Geometry: final body of the model. Coordinates: model frame, mm. Coordinates: 2 decimals unless noted, no trailing zeros. Order: outer loops, then holes, each group sorted by start corner. A loop starts at its lowest first (then second) coordinate and runs counter-clockwise, first axis right, second up. Notation, with made-up numbers: (79.25, 75) -> (124.25, 75) arc R13 ccw to (124.25, 84) -> close; hole circle Ø10 at (51, 40). An arc over 180 degrees is marked (long way). Answer in a Markdown table with one row per item. Add a question column.
1) Section query D-D on z = -3.5. Return the cut outline in (x, y) (3 decimals), then the cut area to 3 significant figures.
2) Ray query, line 1 (X direction, y = 2.9, z = 67); line 2 (Z direction, x = -2, y = 1.8); line 3 (Z direction, x = 25, y = 2.1). Return the intervals inside material, ascending. Write a range as from..to.
3) Section query B-B on x = 15. Return the cut outline in (y, z).
4) Section query C-C on x = 25. Return the cut outline in (y, z).
5) Section query A-A on z = -70. Return the cut outline in (x, y).
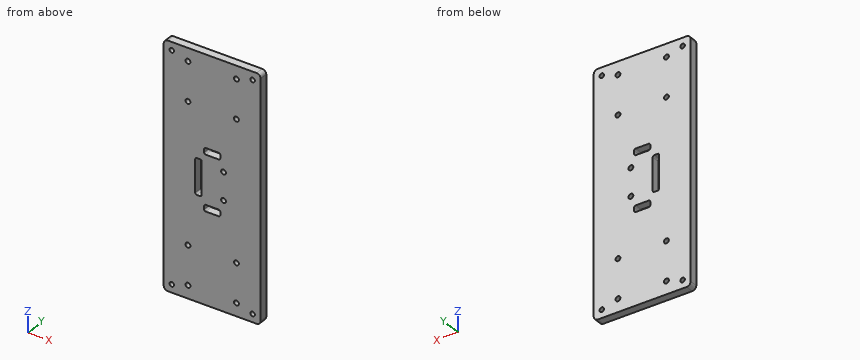
Autodesk Inventor part; units mm, degrees
ref_plane "YZ Plane" through (0, 0, 0) normal (1, 0, 0) x (0, 1, 0)
ref_plane "XZ Plane" through (0, 0, 0) normal (0, 1, 0) x (-1, 0, 0)
ref_plane "XY Plane" through (0, 0, 0) normal (0, 0, 1) x (1, 0, 0)
sketch "Sketch1" plane through (0, 0, 0) normal (0, 1, 0) x (-1, 0, 0)
  line L0 (-30, 75) -> (30, 75)
  line L1 (30, 75) -> (30, -75)
  line L2 (30, -75) -> (-30, -75)
  line L3 (-30, -75) -> (-30, 75)
  line L4 (30, 75) -> (25, 75)
  line L5 (25, 75) -> (25, 70)
  line L6 (25, 70) -> (30, 70)
  line L7 (30, 70) -> (30, 75)
  line L8 (-30, 75) -> (-25, 75)
  line L9 (-25, 75) -> (-25, 70)
  line L10 (-25, 70) -> (-30, 70)
  line L11 (-30, 70) -> (-30, 75)
  line L12 (30, -75) -> (25, -75)
  line L13 (25, -75) -> (25, -70)
  line L14 (25, -70) -> (30, -70)
  line L15 (30, -70) -> (30, -75)
  line L16 (-30, -75) -> (-25, -75)
  line L17 (-25, -75) -> (-25, -70)
  line L18 (-25, -70) -> (-30, -70)
  line L19 (-30, -70) -> (-30, -75)
  circle A0 centre (25, 70) radius 1.4
  circle A1 centre (-25, 70) radius 1.4
  circle A2 centre (25, -70) radius 1.4
  circle A3 centre (-25, -70) radius 1.4
  line L20 (0, 75) -> (13, 75)
  line L21 (0, 75) -> (-13, 75)
  line L22 (-9.515, 11.025) -> (9.515, 11.025)
  line L23 (9.515, 11.025) -> (9.515, -11.025)
  line L24 (9.515, -11.025) -> (-9.515, -11.025)
  line L25 (-9.515, -11.025) -> (-9.515, 11.025)
  line L26 (-9.515, 11.025) -> (9.515, -11.025) construction
  line L27 (9.515, 11.025) -> (-9.515, -11.025) construction
  line L28 (-9.515, -11.025) -> (-7.015, -11.025)
  line L29 (-7.015, -11.025) -> (-7.015, -8.525)
  line L30 (-7.015, -8.525) -> (-9.515, -8.525)
  line L31 (-9.515, -8.525) -> (-9.515, -11.025)
  line L32 (-9.515, 11.025) -> (-7.015, 11.025)
  line L33 (-7.015, 11.025) -> (-7.015, 8.525)
  line L34 (-7.015, 8.525) -> (-9.515, 8.525)
  line L35 (-9.515, 8.525) -> (-9.515, 11.025)
  circle A4 centre (-7.015, 8.525) radius 1.5
  circle A5 centre (-7.015, -8.525) radius 1.5
  line L36 (9.515, 0) -> (8.515, 0)
  line L37 (6.515, -11.025) -> (10.515, -11.025)
  line L38 (10.515, -11.025) -> (10.515, 11.025)
  line L39 (10.515, 11.025) -> (6.515, 11.025)
  line L40 (6.515, 11.025) -> (6.515, -11.025)
  line L41 (6.515, -11.025) -> (10.515, 11.025) construction
  line L42 (10.515, -11.025) -> (6.515, 11.025) construction
  line L43 (0, -75) -> (-20, -75)
  line L44 (-20, -75) -> (-20, -35)
  line L45 (-20, -35) -> (0, -35)
  line L46 (0, -35) -> (0, -75)
  line L47 (0, -75) -> (20, -75)
  line L48 (20, -75) -> (20, -35)
  line L49 (20, -35) -> (0, -35)
  line L50 (0, -35) -> (0, -75)
  line L51 (0, 75) -> (-20, 75)
  line L52 (-20, 75) -> (-20, 35)
  line L53 (-20, 35) -> (0, 35)
  line L54 (0, 35) -> (0, 75)
  line L55 (0, 35) -> (20, 35)
  line L56 (20, 35) -> (20, 75)
  line L57 (20, 75) -> (0, 75)
  line L58 (0, 75) -> (0, 35)
  line L59 (-20, -35) -> (20, -35)
  line L60 (20, -35) -> (20, -43)
  line L61 (20, -43) -> (-20, -43)
  line L62 (-20, -43) -> (-20, -35)
  line L63 (-20, 35) -> (20, 35)
  line L64 (20, 35) -> (20, 43)
  line L65 (20, 43) -> (-20, 43)
  line L66 (-20, 43) -> (-20, 35)
  line L67 (-20, 43) -> (-15, 43)
  line L68 (-15, 43) -> (15, 43)
  line L69 (15, 43) -> (15, 67)
  line L70 (15, 67) -> (-15, 67)
  line L71 (-15, 67) -> (-15, 43)
  line L72 (0, -43) -> (-15, -43)
  line L73 (15, -43) -> (15, -67)
  line L74 (15, -67) -> (-15, -67)
  line L75 (-15, -67) -> (-15, -43)
  circle A6 centre (-15, -67) radius 1.5
  circle A7 centre (15, -67) radius 1.5
  circle A8 centre (-15, -43) radius 1.5
  circle A9 centre (15, -43) radius 1.5
  circle A10 centre (-15, 67) radius 1.5
  circle A11 centre (-15, 43) radius 1.5
  circle A12 centre (15, 43) radius 1.5
  circle A13 centre (15, 67) radius 1.5
  line L76 (-20, 35) -> (20, 35)
  line L77 (20, 35) -> (20, 19)
  line L78 (20, 19) -> (-20, 19)
  line L79 (-20, 19) -> (-20, 35)
  line L80 (20, -35) -> (-20, -35)
  line L81 (-20, -35) -> (-20, -19)
  line L82 (-20, -19) -> (20, -19)
  line L83 (20, -19) -> (20, -35)
  line L84 (0, 19) -> (5, 19)
  line L85 (5, 19) -> (5, 15)
  line L86 (5, 15) -> (0, 15)
  line L87 (0, 15) -> (0, 19)
  line L88 (0, 19) -> (-5, 19)
  line L89 (-5, 19) -> (-5, 15)
  line L90 (-5, 15) -> (0, 15)
  line L91 (0, 15) -> (0, 19)
  line L92 (0, -19) -> (5, -19)
  line L93 (5, -19) -> (5, -15)
  line L94 (5, -15) -> (0, -15)
  line L95 (0, -15) -> (0, -19)
  line L96 (0, -15) -> (-5, -15)
  line L97 (-5, -15) -> (-5, -19)
  line L98 (-5, -19) -> (0, -19)
  line L99 (0, -19) -> (0, -15)
  point P0 (0, 0)
  point P1 (6.515, 11.025)
  point P2 (6.515, -11.025)
  point P3 (-5, 19)
  point P4 (5, 19)
  point P5 (0, 15)
  dimension "d0" = 60
  dimension "d1" = 150
  dimension "d2" = 5
  dimension "d3" = 5
  dimension "d4" = 5
  dimension "d5" = 5
  dimension "d6" = 5
  dimension "d7" = 5
  dimension "d8" = 5
  dimension "d9" = 5
  dimension "d10" = 2.8
  dimension "d11" = 2.8
  dimension "d39" = 19.03
  dimension "d40" = 22.05
  dimension "d41" = 2.5
  dimension "d42" = 2.5
  dimension "d43" = 2.5
  dimension "d44" = 2.5
  dimension "d45" = 3
  dimension "d46" = 3
  dimension "d47" = 1
  dimension "d48" = 4
  dimension "d54" = 20
  dimension "d55" = 40
  dimension "d56" = 20
  dimension "d57" = 20
  dimension "d58" = 40
  dimension "d59" = 20
  dimension "d60" = 8
  dimension "d61" = 8
  dimension "d62" = 5
  dimension "d63" = 30
  dimension "d64" = 24
  dimension "d65" = 24
  dimension "d66" = 3
  dimension "d67" = 3
  dimension "d68" = 3
  dimension "d69" = 3
  dimension "d70" = 3
  dimension "d71" = 3
  dimension "d72" = 3
  dimension "d75" = 16
  dimension "d76" = 16
  dimension "d77" = 5
  dimension "d78" = 4
  dimension "d79" = 5
  dimension "d80" = 5
  dimension "d81" = 4
  dimension "d82" = 5
extrude "Extrusion1" add sketch "Sketch1" along normal blind 5 contours L0 L9 A1 L10 L3 | L0 L52 L79 L78 L89 L90 L86 L85 L77 L56 L5 A0 L6 L1 L14 A2 L13 L2 L48 L83 L82 L93 L94 L96 L97 L81 L44 L17 A3 L18 L3 L10 A1 L9 | L0 L54 L70 A10 L71 A11 L65 L52 | L18 A3 L17 L2 L3 | L65 A11 L54 L53 L52 | L0 L56 L65 A12 L69 A13 L70 L54 | L53 L55 L77 L78 L79 | A11 L71 L65 | L65 A11 | L70 A13 L69 A12 L65 L54 | L54 L65 A11 L71 A10 L70 | L54 L65 A12 L56 L55 | L71 A11 L65 | L44 L61 A8 L75 A6 L74 L46 L2 | A13 L69 L70 | L70 L69 A13 | A10 L71 L70 | L70 L71 A10 | L46 L74 A7 L73 A9 L61 L48 L2 | L44 L45 L46 L61 A8 | L0 L1 L6 A0 L5 | A12 L69 L65 | L65 A12 | L74 A6 L75 A8 L61 L46 | L46 L61 A9 L73 A7 L74 | L81 L82 L83 L49 L45 | A8 L61 | L61 L75 A8 | L65 L69 A12 | L13 A2 L14 L1 L2 | L61 A9 L46 L49 L48 | A7 L73 L74 | L74 L73 A7 | A6 L75 L74 | L74 L75 A6 | L61 A8 L75 | A9 L73 L61 | L61 A9 | L61 L73 A9 | L22 L33 A4 L34 L25 | L22 L40 L24 L29 A5 L30 L25 L34 A4 L33 | L30 A5 L29 L24 L25
fillet "Fillet1" radius 2.5 4 edges at (-30, 2.5, 75) (-30, 2.5, -75) (30, 2.5, -75) (30, 2.5, 75)
fillet "Fillet2" radius 1 2 edges at (-6.515, 2.5, 11.025) (-10.515, 2.5, 11.025)
fillet "Fillet3" radius 1 2 edges at (-6.515, 2.5, -11.025) (-10.515, 2.5, -11.025)
extrude "Extrusion2" cut sketch "Sketch1" along normal blind 5 contours A11 L71 L65 | L65 A11 | L71 A11 L65 | A13 L69 L70 | L70 L69 A13 | A10 L71 L70 | L70 L71 A10 | A12 L69 L65 | L65 A12 | A8 L61 | L61 L75 A8 | L65 L69 A12 | A7 L73 L74 | L74 L73 A7 | A6 L75 L74 | L74 L75 A6 | L61 A8 L75 | A9 L73 L61 | L61 A9 | L61 L73 A9
fillet "Fillet4" radius 1 8 edges at (-5, 2.5, -15) (5, 2.5, -15) (5, 2.5, -19) (-5, 2.5, -19) (-5, 2.5, 19) (5, 2.5, 19) (5, 2.5, 15) (-5, 2.5, 15)
properties part number "DeDuoi"
Result:
| question | item | result |
|---|---|---|
| 1 | outline | (-30, 0) -> (-10.515, 0) -> (-10.515, 5) -> (-30, 5) -> close; (-6.515, 0) -> (30, 0) -> (30, 5) -> (-6.515, 5) -> close |
| 1 | area | 280 mm2 |
| 2 | line 1 | -30..-16.5, -13.5..13.5, 16.5..30 |
| 2 | line 2 | -75..-19, -15..15, 19..75 |
| 2 | line 3 | -75..-71.4, -68.6..68.6, 71.4..75 |
| 3 | outline | (0, -75) -> (5, -75) -> (5, -68.5) -> (0, -68.5) -> close; (0, -65.5) -> (5, -65.5) -> (5, -44.5) -> (0, -44.5) -> close; (0, -41.5) -> (5, -41.5) -> (5, 41.5) -> (0, 41.5) -> close; (0, 44.5) -> (5, 44.5) -> (5, 65.5) -> (0, 65.5) -> close; (0, 68.5) -> (5, 68.5) -> (5, 75) -> (0, 75) -> close |
| 4 | outline | (0, -75) -> (5, -75) -> (5, -71.4) -> (0, -71.4) -> close; (0, -68.6) -> (5, -68.6) -> (5, 68.6) -> (0, 68.6) -> close; (0, 71.4) -> (5, 71.4) -> (5, 75) -> (0, 75) -> close |
| 5 | outline | (-30, 0) -> (-26.4, 0) -> (-26.4, 5) -> (-30, 5) -> close; (-23.6, 0) -> (23.6, 0) -> (23.6, 5) -> (-23.6, 5) -> close; (26.4, 0) -> (30, 0) -> (30, 5) -> (26.4, 5) -> close |
